```python
from build123d import *

# Parameters (mm, degrees)
SKETCH_1_W                = 15
SKETCH_1_H                = 15
SKETCH_1_W_2              = 12
SKETCH_1_H_2              = 12
EXTRUDE_1_DEPTH           = 167.65
CUT_EXTRUDE_1_OUTLINE_R   = 1.5
CUT_EXTRUDE_1_OUTLINE_R_2 = 1.6
CUT_EXTRUDE_1_DEPTH       = 15


# Read off the part's stored shape, not the designer's step: 切除-拉伸1
with BuildPart() as part:
    # 草图1 → 凸台-拉伸1 (new body)
    with BuildSketch(Plane(origin=(0, 0, 0), x_dir=(1, 0, 0), z_dir=(0, 1, 0))):
        with Locations((7.5, 7.5)):
            Rectangle(SKETCH_1_W, SKETCH_1_H)
        with Locations((7.5, 7.5)):
            Rectangle(SKETCH_1_W_2, SKETCH_1_H_2, mode=Mode.SUBTRACT)
    extrude(amount=EXTRUDE_1_DEPTH)

    # 切除-拉伸1 outline → 切除-拉伸1 (cut)
    with BuildSketch(Plane.YZ):
        with Locations((12.5, -7.5)):
            Circle(CUT_EXTRUDE_1_OUTLINE_R)
        with Locations((32.5, -7.5)):
            Circle(CUT_EXTRUDE_1_OUTLINE_R)
        with Locations((54.975, -7.5)):
            Circle(CUT_EXTRUDE_1_OUTLINE_R_2)
        with Locations((83.825, -7.5)):
            Circle(CUT_EXTRUDE_1_OUTLINE_R_2)
        with Locations((112.675, -7.5)):
            Circle(CUT_EXTRUDE_1_OUTLINE_R_2)
        with Locations((135.15, -7.5)):
            Circle(CUT_EXTRUDE_1_OUTLINE_R)
        with Locations((155.15, -7.5)):
            Circle(CUT_EXTRUDE_1_OUTLINE_R)
    extrude(amount=CUT_EXTRUDE_1_DEPTH, mode=Mode.SUBTRACT)


solid = part.part
```
Geometry: final body of the model. Coordinates: model frame, mm. A direction names the side the tool comes from. Round coordinates to 2 decimals unless told otherwise and drop trailing zeros. Order: outer loops, then holes, each group sorted by start corner. A loop starts at its lowest first (then second) coordinate and runs counter-clockwise, first axis right, second up. Notation, with made-up numbers: (62, 87) - (106, 87) arc R9 ccw to (106, 93) - close; hole circle Ø9 at (-32.75, 53). An arc over 180 degrees is marked (long way). Write item = value, one per line. Start each with the question number.
Q1. Cut plane B-B on y = 94. Return the cut outline in (x, z).
Q2. Pull-direction query (Y, two-part tool) for faces 3 (the flat face through (14, 167.65, -8)), 4 (the flat face through (7, 83, -13.5)), 5 (the cylindrical face through (14.24, 82.555, -8.474)); classes: +Y half, -Y half, draft (parallel to the pull), parting line (faces both ways), or undercut.
Q3. Access query for faces 1 (the flat face through (13.5, 82.7, -6.1)), 2 (the flat face through (15, 82.7, -5.7)). Directions: +Z, -Z, +X, -X, +Y, -Y. A direction counts if a zero-diameter tool reaches every point of the face in a straight line with its end or side. Return the directions, or none.
Q4. Pin query (flat end, axial travel): pin 1 (2 mm diameter, centred on x = 3, z = -5.5, fed in from +Y). Return the tip coordinate at first contact, or that it passes through.
Q5. Ray query, line 1 (Z direction, x = 14.6, y = 135.15); line 2 (Z direction, x = 6, y = 125.5); line 3 (X direction, y = 112, z = -4.5). Return the intervals inside material, ascending. Write a range as from..to.
Q6. Cut plane C-C on z = -4.25. Return the cut outline in (x, y).
Q7. Cut plane A-A on x = 3.5. Return the cut outline in (y, z), and give its area (3 significant figures).
Q8. Cut plane D-D on y = 135.15. Return the cut outline in (x, z).
Outcome:
q1.outline = (0, -15) - (15, -15) - (15, 0) - (0, 0) - close; hole (1.5, -13.5) - (13.5, -13.5) - (13.5, -1.5) - (1.5, -1.5) - close
q2.face_3 = +Y half
q2.face_4 = draft
q2.face_5 = undercut
q3.face_1 = +Y, -Y
q3.face_2 = +Z, -Z, +X, +Y, -Y
q4.pin_1 = through
q5.line_1 = -15..-9, -6..0
q5.line_2 = -15..-13.5, -1.5..0
q5.line_3 = 0..1.5, 13.5..15
q6.outline = (0, 0) - (1.5, 0) - (1.5, 167.65) - (0, 167.65) - close; (13.5, 0) - (15, 0) - (15, 167.65) - (13.5, 167.65) - close
q7.outline = (0, -15) - (167.65, -15) - (167.65, -13.5) - (0, -13.5) - close; (0, -1.5) - (167.65, -1.5) - (167.65, 0) - (0, 0) - close
q7.area = 503 mm^2
q8.outline = (0, -15) - (15, -15) - (15, -9) - (13.5, -9) - (13.5, -13.5) - (1.5, -13.5) - (1.5, -9) - (0, -9) - close; (0, -6) - (1.5, -6) - (1.5, -1.5) - (13.5, -1.5) - (13.5, -6) - (15, -6) - (15, 0) - (0, 0) - close
